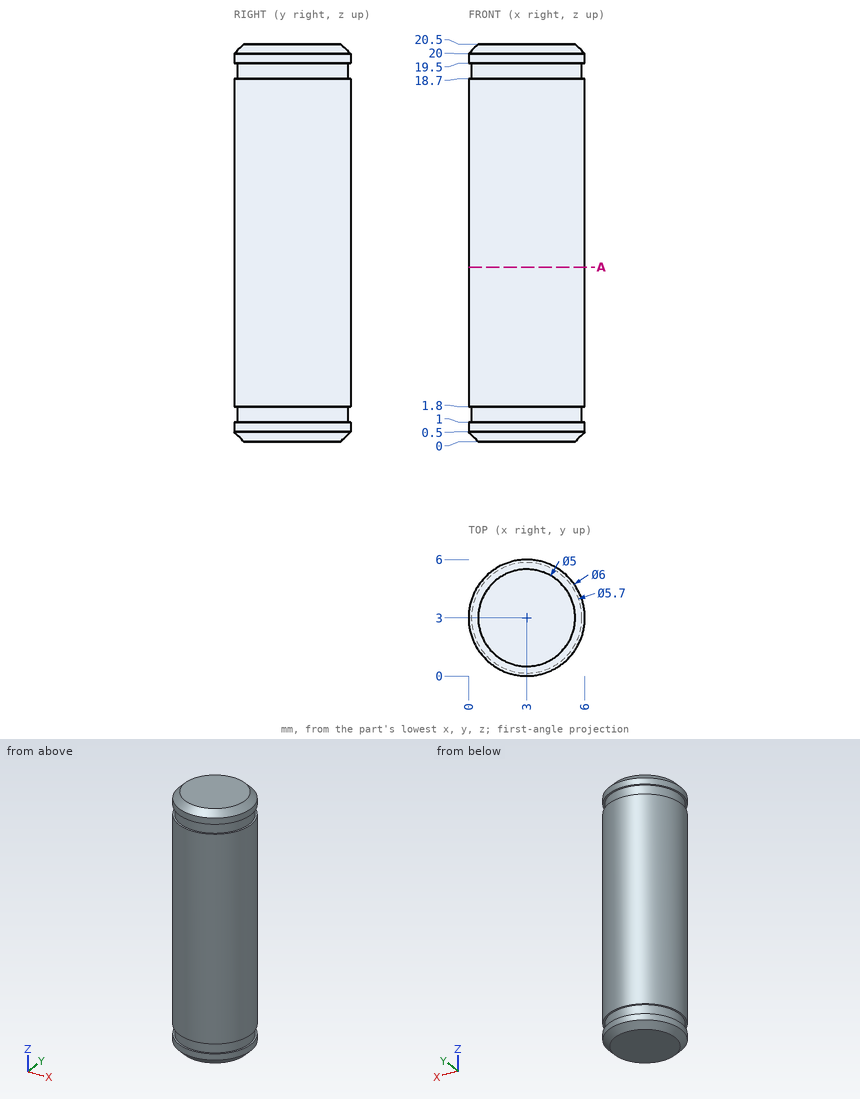
Can you work these out from the drawing? Everything is in mm from the part's minimum corner. Round coordinates to 2 decimals unless told otherwise and drop trailing zeros. Order: outer loops, then holes, each group sorted by start corner. A loop starts at its lowest first (then second) coordinate and runs counter-clockwise, first axis right, second up. Notation, with made-up numbers: (-23, 16) -> (-11, 16) arc R34 cw to (-11, 47) -> close; hole circle Ø3 at (-31, 55.25). An arc over 180 degrees is marked (long way). Return JSON: item names as keys, results as strings. Group by question number.
1. I need wall thicknesses on line 1 (Z direction, x = 1.5, y = 5.5); line 2 (X direction, y = 3.6, z = 3.75); line 3 (Y direction, x = 4.9, z = 7.75). Which ranges of each line are inside material? Lowest first, please. Write a range as [from, to].
2. Will this pin go through, and if not, where does the flat tip stop? pin 1 (2 mm diameter, centred on y = 3.5, z = 9.5, fed in from +X).
3. If we section it at A-A, the plane z = 9: Write out the boundary of the cut face in (x, y).
Output values:
{
 "1": {"line 1": "[0.42, 1], [1.8, 18.7], [19.5, 20.08]", "line 2": "[0.06, 5.94]", "line 3": "[0.68, 5.32]"},
 "2": {"pin 1": "x = 6"},
 "3": {"outline": "circle Ø6 at (3, 3)"}
}
